Check sheet for the modelled part. Datum: model origin and axes. Units: mm. Round coordinates to 2 decimals unless told otherwise and drop trailing zeros. Order: outer loops, then holes, each group sorted by start corner. A loop starts at its lowest first (then second) coordinate and runs counter-clockwise, first axis right, second up. Notation, with made-up numbers: (-35.75, 54.5) -> (-14.75, 54.5) arc R21 ccw to (-14.75, 81.5) -> close; hole circle Ø8 at (51, -23.75). An arc over 180 degrees is marked (long way). Answer in a Markdown table with one row per item.
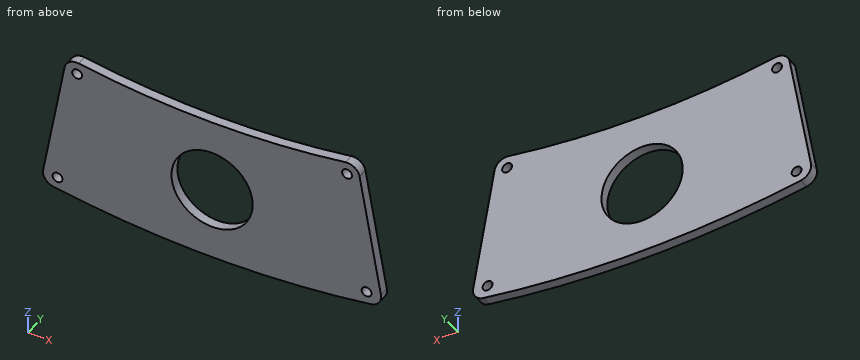
from build123d import *

# Parameters (mm, degrees)
SKETCH_1_R             = 16.5
SM_BASE_FLANGE_1_DEPTH = 4
SKETCH_4_R             = 2
CUT_EXTRUDE_1_DEPTH    = 10
FILLET_3_R             = 5


# Sheet-metal steps are written as plain solids
with BuildPart() as part:
    # Sketch 1 → Базовая кромка1 (new body)
    with BuildSketch(Plane(origin=(0, 0, 0), x_dir=(1, 0, 0), z_dir=(0, 1, 0))):
        with BuildLine():
            Line((-59.040380407, 334.834636024), (-69.459271067, 393.923101205))
            ThreePointArc((-69.459271067, 393.923101205), (0, 400), (69.459271067, 393.923101205))
            Line((69.459271067, 393.923101205), (59.040380407, 334.834636024))
            ThreePointArc((59.040380407, 334.834636024), (0, 340), (-59.040380407, 334.834636024))
        make_face()
        with Locations(Location((0, 370, 0), (0, 0, 270))):
            Circle(SKETCH_1_R, mode=Mode.SUBTRACT)
    extrude(amount=-SM_BASE_FLANGE_1_DEPTH)

    # Эскиз4 → Вырез-Вытянуть1 (cut)
    with BuildSketch(Plane(origin=(0, 0, 0), x_dir=(1, 0, 0), z_dir=(0, 1, 0))):
        with Locations(Location((62.748327317, 389.984163036, 0), (0, 0, 270))):
            Circle(SKETCH_4_R)
        with Locations(Location((54.805501074, 340.619079107, 0), (0, 0, 270))):
            Circle(SKETCH_4_R)
        with Locations(Location((-54.805501074, 340.619079107, 0), (0, 0, 270))):
            Circle(SKETCH_4_R)
        with Locations(Location((-62.748327317, 389.984163036, 0), (0, 0, 270))):
            Circle(SKETCH_4_R)
    extrude(amount=-CUT_EXTRUDE_1_DEPTH, mode=Mode.SUBTRACT)

    # Скругление3
    fillet_3_edges = [part.edges().sort_by_distance(p)[0] for p in [
        (-59.040380407, -2, -334.834636024),
        (-69.459271067, -2, -393.923101205),
        (69.459271067, -2, -393.923101205),
        (59.040380407, -2, -334.834636024),
    ]]
    fillet(fillet_3_edges, radius=FILLET_3_R)


solid = part.part
Item 1: Depth check by flat-ended pin: P1, Ø2, axis at y = -3, z = -383, coming from the +X side; P2, Ø1, axis at y = -1, z = -373.5, coming from the -X side; P3, Ø20, axis at x = 0, z = -370, coming from the -Y side; P4, Ø1.5, axis at x = -4, y = -3.5, coming from the +Z side. Enter the tip coordinate at first touch or a pass-through.
Result sheet:
| item | result |
|---|---|
| P1 | stops at x = 67.71 |
| P2 | stops at x = -65.95 |
| P3 | passes through |
| P4 | stops at z = -339.97 |
Item 2: Scan lines: line 1 (X direction, y = -3.15, z = -389); line 2 (X direction, y = -0.7, z = -391); line 3 (X direction, y = -2.15, z = -370). Record each from-to range of solid material in increasing order. Write a range as [from, to].
Result sheet:
| item | result |
|---|---|
| line 1 | x = [-68.59, -64.49], [-61.01, 61.01], [64.49, 68.59] |
| line 2 | x = [-68.52, -64.47], [-61.03, 61.03], [64.47, 68.52] |
| line 3 | x = [-65.24, -16.5], [16.5, 65.24] |
Item 3: Cross-section at A-A (x = 0). Record the boundary of the cut face in (y, z), and give its area (3 significant figures).
Result sheet:
| item | result |
|---|---|
| outline | (-4, -400) -> (0, -400) -> (0, -386.5) -> (-4, -386.5) -> close; (-4, -353.5) -> (0, -353.5) -> (0, -340) -> (-4, -340) -> close |
| area | 108 mm^2 |
Item 4: Cross-section at B-B (y = -2.25). Record the boundary of the cut face in (x, z).
Result sheet:
| item | result |
|---|---|
| outline | (-68.59, -388.97) arc R5 ccw to (-64.47, -394.77) arc R400 ccw to (64.47, -394.77) arc R5 ccw to (68.59, -388.97) -> (59.9, -339.72) arc R5 ccw to (54.18, -335.66) arc R340 cw to (-54.18, -335.66) arc R5 ccw to (-59.9, -339.72) -> close; hole circle Ø4 at (-62.75, -389.98); hole circle Ø4 at (-54.81, -340.62); hole circle Ø33 at (0, -370); hole circle Ø4 at (54.81, -340.62); hole circle Ø4 at (62.75, -389.98) |
Item 5: Cross-section at C-C (z = -370). Record the boundary of the cut face in (x, y).
Result sheet:
| item | result |
|---|---|
| outline | (-65.24, -4) -> (-16.5, -4) -> (-16.5, 0) -> (-65.24, 0) -> close; (16.5, -4) -> (65.24, -4) -> (65.24, 0) -> (16.5, 0) -> close |
Item 6: Cross-section at D-D (x = -19.5). Record the boundary of the cut face in (y, z), and give its area (3 significant figures).
Result sheet:
| item | result |
|---|---|
| outline | (-4, -399.52) -> (0, -399.52) -> (0, -339.44) -> (-4, -339.44) -> close |
| area | 240 mm^2 |
